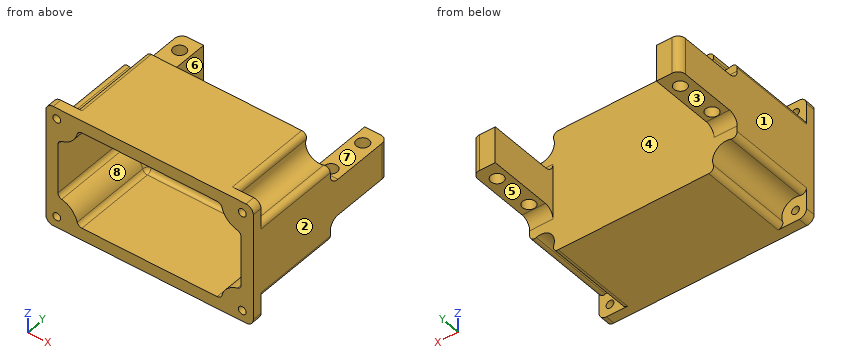
```python
from build123d import *

# Parameters (mm, degrees)
EXTRUDE_1_DEPTH     = 40
SKETCH_2_W          = 9.5
SKETCH_2_H          = 30
EXTRUDE_2_DEPTH     = 15
SKETCH_3_R          = 2.6
CUT_EXTRUDE_1_DEPTH = 89.290712988
FILLET_1_R          = 3
FILLET_2_R          = 4
SKETCH_4_R          = 1.6
CUT_EXTRUDE_2_DEPTH = 64.492125496
CUT_EXTRUDE_3_DEPTH = 36
FILLET_3_R          = 2
SKETCH_7_R          = 5.6
CUT_EXTRUDE_4_DEPTH = 36
FILLET_4_R          = 2


with BuildPart() as part:
    # 草图1 → 凸台-拉伸1 (new body)
    with BuildSketch(Plane(origin=(0, 0, 0), x_dir=(1, 0, 0), z_dir=(0, 1, 0))):
        with BuildLine():
            Line((-39.5, -25), (39.5, -25))
            ThreePointArc((39.5, -25), (41.621320344, -24.121320344), (42.5, -22))
            Line((42.5, -22), (42.5, 22))
            ThreePointArc((42.5, 22), (41.621320344, 24.121320344), (39.5, 25))
            Line((39.5, 25), (-39.5, 25))
            ThreePointArc((-39.5, 25), (-41.621320344, 24.121320344), (-42.5, 22))
            Line((-42.5, 22), (-42.5, -22))
            ThreePointArc((-42.5, -22), (-41.621320344, -24.121320344), (-39.5, -25))
        make_face()
    extrude(amount=EXTRUDE_1_DEPTH)

    # 草图2 → 凸台-拉伸2 (add)
    with BuildSketch(Plane.XY.offset(-7)):
        with Locations((-37.75, 55)):
            Rectangle(SKETCH_2_W, SKETCH_2_H)
    extrude_2 = extrude(amount=EXTRUDE_2_DEPTH)

    # 镜向1: 凸台-拉伸2 across plane
    add(extrude_2.mirror(Plane(origin=(0, 0, 0), x_dir=(0, 0, 1), z_dir=(1, 0, 0))))

    # 草图3 → 切除-拉伸1 (cut, through all)
    with BuildSketch(Plane.XY.offset(8)):
        with Locations((37.5, 63.25)):
            Circle(SKETCH_3_R)
        with Locations((37.5, 46.75)):
            Circle(SKETCH_3_R)
        with Locations((-37.5, 63.25)):
            Circle(SKETCH_3_R)
        with Locations((-37.5, 46.75)):
            Circle(SKETCH_3_R)
    extrude(amount=-CUT_EXTRUDE_1_DEPTH, mode=Mode.SUBTRACT)

    # 圆角1
    fillet_1_edges = [part.edges().sort_by_distance(p)[0] for p in [
        (-42.5, 70, 0.5),
        (42.5, 70, 0.5),
    ]]
    fillet(fillet_1_edges, radius=FILLET_1_R)

    # 圆角2
    fillet_2_edges = [part.edges().sort_by_distance(p)[0] for p in [
        (-37.75, 40, -7),
        (-37.75, 40, 8),
        (37.75, 40, 8),
        (37.75, 40, -7),
    ]]
    fillet(fillet_2_edges, radius=FILLET_2_R)

    # 草图4 → 切除-拉伸2 (cut, through all)
    with BuildSketch(Plane(origin=(0, 40, 0), x_dir=(1, 0, 0), z_dir=(0, 1, 0))):
        with Locations(Location((-38, 20.5, 0), (0, 0, 270))):
            Circle(SKETCH_4_R)
        with Locations(Location((38, 20.5, 0), (0, 0, 270))):
            Circle(SKETCH_4_R)
        with Locations(Location((38, -20.5, 0), (0, 0, 270))):
            Circle(SKETCH_4_R)
        with Locations(Location((-38, -20.5, 0), (0, 0, 270))):
            Circle(SKETCH_4_R)
    extrude(amount=-CUT_EXTRUDE_2_DEPTH, mode=Mode.SUBTRACT)

    # 草图5 → 切除-拉伸3 (cut)
    with BuildSketch(Plane.XZ):
        with BuildLine():
            ThreePointArc((29.414547187, -20), (31.918881682, -14.418881682), (37.5, -11.914547187))
            Line((37.5, -11.914547187), (37.5, 11.914547187))
            ThreePointArc((37.5, 11.914547187), (31.918881682, 14.418881682), (29.414547187, 20))
            Line((29.414547187, 20), (-29.414547187, 20))
            ThreePointArc((-29.414547187, 20), (-31.918881682, 14.418881682), (-37.5, 11.914547187))
            Line((-37.5, 11.914547187), (-37.5, -11.914547187))
            ThreePointArc((-37.5, -11.914547187), (-31.918881682, -14.418881682), (-29.414547187, -20))
            Line((-29.414547187, -20), (29.414547187, -20))
        make_face()
    extrude(amount=-CUT_EXTRUDE_3_DEPTH, mode=Mode.SUBTRACT)

    # 圆角3
    fillet_3_edges = [part.edges().sort_by_distance(p)[0] for p in [
        (31.918881682, 36, -14.418881682),
        (-31.918881682, 36, -14.418881682),
        (-31.918881682, 36, 14.418881682),
        (31.918881682, 36, 14.418881682),
        (37.5, 36, 0),
        (37.5, 18, 11.914547187),
        (29.414547187, 18, 20),
        (0, 36, 20),
        (-29.414547187, 18, 20),
        (-37.5, 18, 11.914547187),
        (-37.5, 36, 0),
        (-37.5, 18, -11.914547187),
        (-29.414547187, 18, -20),
        (0, 36, -20),
        (29.414547187, 18, -20),
        (37.5, 18, -11.914547187),
    ]]
    fillet(fillet_3_edges, radius=FILLET_3_R)

    # 草图7 → 切除-拉伸4 (cut)
    with BuildSketch(Plane(origin=(0, 40, 0), x_dir=(1, 0, 0), z_dir=(0, 1, 0))):
        with Locations((-38, 20.5)):
            Circle(SKETCH_7_R)
        with Locations((38, 20.5)):
            Circle(SKETCH_7_R)
        with Locations((-38, -20.5)):
            Circle(SKETCH_7_R)
        with Locations((38, -20.5)):
            Circle(SKETCH_7_R)
    extrude(amount=-CUT_EXTRUDE_4_DEPTH, mode=Mode.SUBTRACT)

    # 圆角4
    fillet_4_edges = [part.edges().sort_by_distance(p)[0] for p in [
        (-34.666833338, 22, 25),
        (34.666833338, 22, 25),
        (-42.5, 22, -17.166833338),
        (34.666833338, 22, -25),
        (-34.666833338, 22, -25),
        (42.5, 22, -17.166833338),
        (42.5, 22, 17.166833338),
        (-42.5, 22, 17.166833338),
    ]]
    fillet(fillet_4_edges, radius=FILLET_4_R)


solid = part.part
```
Check sheet for the modelled part. Datum: model origin and axes. Units: mm. Face numbers are marked on the shaded views. A direction names the side the tool comes from. Round coordinates to 2 decimals unless told otherwise and drop trailing zeros. Order: outer loops, then holes, each group sorted by start corner. A loop starts at its lowest first (then second) coordinate and runs counter-clockwise, first axis right, second up. Notation, with made-up numbers: (39.5, 79.5) - (44.5, 79.5) arc R28 ccw to (44.5, 107.5) - close; hole circle Ø2 at (51, 63). An arc over 180 degrees is marked (long way). Answer as CSV lines item,"result". Start each with the question number.
1) Draft check along X on the marked faces 1, 2, 3 and 4. Enter one of: +X half, -X half, draft (parallel to the pull), parting line (faces both ways), or undercut.
2) Tool access check on the marked faces 5, 6, 7 and 8. Record the directions out of +Z, -Z, +X, -X, +Y, -Y that give a thin tool (end or side, any length) a straight path to the whole face; none if there is none.
3) Depth check by flat-ended pin: pin 1 (1.5 mm diameter, centred on y = 16.5, z = -15.5, fed in from -X); pin 2 (7.5 mm diameter, centred on x = 37.5, y = 56.5, fed in from -Z); pin 3 (3 mm diameter, centred on x = -38, z = 20.5, fed in from -Y); pin 4 (8 mm diameter, centred on x = -11, z = -13, fed in from +Y). Enter the tip coordinate at first touch or a pass-through.
4) Section check C-C (z = 0.5). Record the cut outline in (x, y), then the cut area to 3 significant figures.
5) Section check A-A (y = 59). Record the cut outline in (x, z), then the cut area to 3 significant figures.
6) Section check B-B (y = 46.75). Record the cut outline in (x, z), then the cut area to 3 significant figures.
7) Section check D-D (x = -1). Record the cut outline in (y, z), then the cut area to 3 significant figures.
8) Scan lines: probe 1 along X at (y, z) = (1.4, -20.5); probe 2 along Z at (x, y) = (-8, 15); probe 3 along X at (y, z) = (23, 2). Record each from-to range of solid material in increasing order.
Determined:
1,face 1,"-X half"
1,face 2,"+X half"
1,face 3,"draft"
1,face 4,"undercut"
2,face 5,"-Z, +X, -X, +Y"
2,face 6,"+Z, -Z, +Y"
2,face 7,"+Z, +X, -X, +Y"
2,face 8,"-Y"
3,pin 1,"x = -41.9"
3,pin 2,"z = -7"
3,pin 3,"through"
3,pin 4,"y = 40"
4,outline,"(-42.5, 0) - (-37.5, 0) - (-37.5, 34) arc R2 cw to (-35.5, 36) - (35.5, 36) arc R2 cw to (37.5, 34) - (37.5, 0) - (42.5, 0) - (42.5, 67) arc R3 ccw to (39.5, 70) - (33, 70) - (33, 40) - (-33, 40) - (-33, 70) - (-39.5, 70) arc R3 ccw to (-42.5, 67) - close; hole circle Ø5.2 at (-37.5, 46.75); hole circle Ø5.2 at (-37.5, 63.25); hole circle Ø5.2 at (37.5, 46.75); hole circle Ø5.2 at (37.5, 63.25)"
4,area,"1,180 mm^2"
5,outline,"(-42.5, -7) - (-33, -7) - (-33, 8) - (-42.5, 8) - close; (33, -7) - (42.5, -7) - (42.5, 8) - (33, 8) - close"
5,area,"285 mm^2"
6,outline,"(-42.5, -7) - (-40.1, -7) - (-40.1, 8) - (-42.5, 8) - close; (-34.9, -7) - (-33, -7) - (-33, 8) - (-34.9, 8) - close; (33, -7) - (34.9, -7) - (34.9, 8) - (33, 8) - close; (40.1, -7) - (42.5, -7) - (42.5, 8) - (40.1, 8) - close"
6,area,"129 mm^2"
7,outline,"(0, -25) - (40, -25) - (40, 25) - (0, 25) - (0, 20) - (34, 20) arc R2 cw to (36, 18) - (36, -18) arc R2 cw to (34, -20) - (0, -20) - close"
7,area,"562 mm^2"
8,probe 1,"-42.5 to -39.6, -36.4 to 36.4, 39.6 to 42.5"
8,probe 2,"-25 to -20, 20 to 25"
8,probe 3,"-42.5 to -37.5, 37.5 to 42.5"
